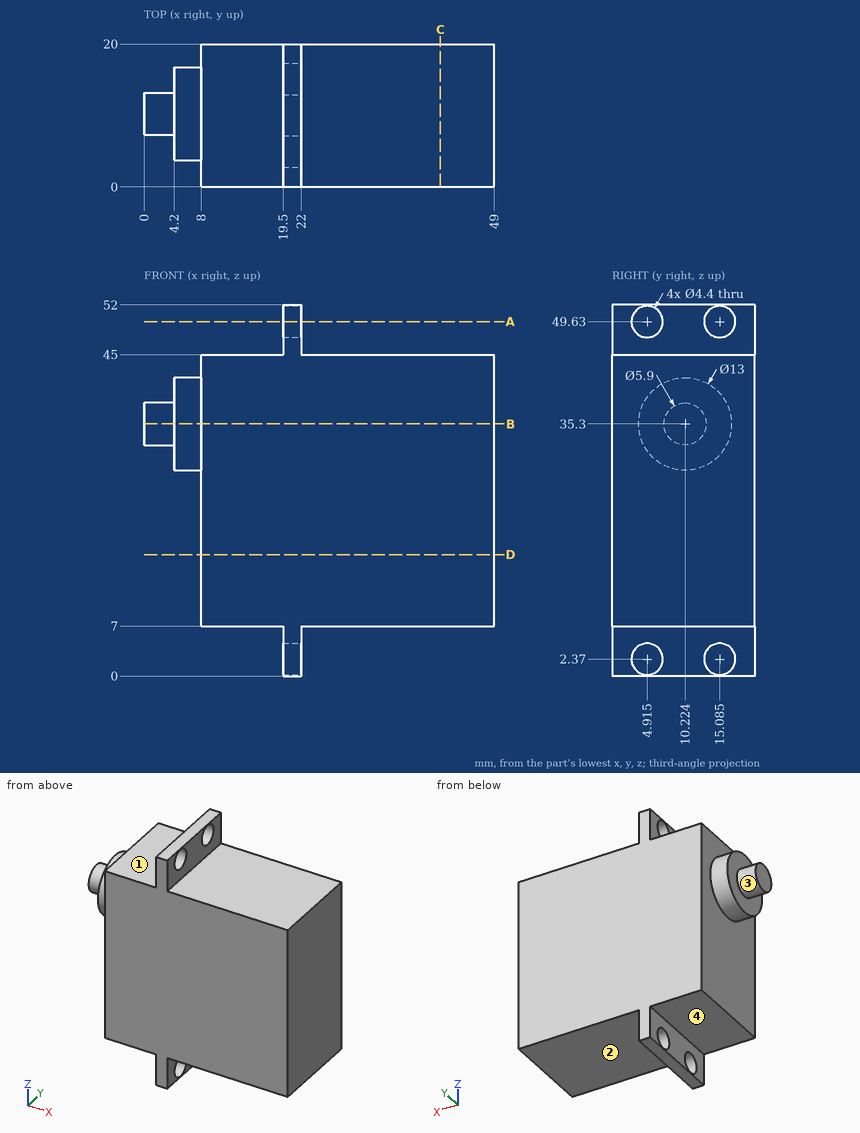
Check sheet for the drawn part. Datum: minimum x, y, z corner. Units: mm. A direction names the side the tool comes from. Round coordinates to 2 decimals unless told otherwise and drop trailing zeros. Order: outer loops, then holes, each group sorted by start corner. A loop starts at its lowest first (then second) coordinate and runs counter-clockwise, first axis right, second up.
(1) Scan lines: probe 1 along Y at (x, z) = (21.3, 2.37) (1 decimal); probe 2 along X at (y, z) = (18.25, 47); probe 3 along Z at (x, y) = (45.5, 17). Record each from-to range of solid material in increasing order.
(2) Go/stop test with flat-tipped pins: P1, Ø2, axis at y = 11.5, z = 26, coming from the -X side; P2, Ø3.5, axis at y = 6.5, z = 2.5, coming from the +X side; P3, Ø12, axis at x = 39.5, y = 3.5, coming from the +Z side; P4, Ø3.5, axis at y = 4.915, z = 49.63, coming from the +X side. Record where each tip stops, or that it passes through.
(3) Cross-section at C-C, the plane x = 41.5. Enter the section's corners in (y, z).
(4) Access from +Z, -Z, +X, -X, +Y, -Y to the whole of each face (thin tool, end or side, straight path). Record for the marked faces 1, 2, 3 and 4.
(5) Cross-section at B-B, the plane z = 35.3. Enter the section's corners in (x, y) (1 decimal), and give its area (3 significant figures).
(6) Cross-section at D-D, the plane z = 17. Enter the section's corners in (x, y).
(7) Cross-section at A-A, the plane z = 49.63. Enter the section's corners in (x, y) (1 decimal), and give its area (3 significant figures).
Check sheet entries:
1. probe 1: y = 0 to 2.7, 7.1 to 12.9, 17.3 to 20
1. probe 2: x = 19.5 to 22
1. probe 3: z = 7 to 45
2. P1: stops at x = 8
2. P2: stops at x = 22
2. P3: stops at z = 45
2. P4: passes through
3. outline: (0, 7) - (20, 7) - (20, 45) - (0, 45) - close
4. face 1: +Z, -X, +Y, -Y
4. face 2: -Z, +X, +Y, -Y
4. face 3: -X
4. face 4: -Z, -X, +Y, -Y
5. outline: (0, 7.3) - (4.2, 7.3) - (4.2, 3.7) - (8, 3.7) - (8, 0) - (49, 0) - (49, 20) - (8, 20) - (8, 16.7) - (4.2, 16.7) - (4.2, 13.2) - (0, 13.2) - close
5. area: 894 mm2
6. outline: (8, 0) - (49, 0) - (49, 20) - (8, 20) - close
7. outline: (19.5, 0) - (22, 0) - (22, 2.7) - (19.5, 2.7) - close; (19.5, 7.1) - (22, 7.1) - (22, 12.9) - (19.5, 12.9) - close; (19.5, 17.3) - (22, 17.3) - (22, 20) - (19.5, 20) - close
7. area: 28.0 mm2
